Verification items for the finished model (mm, model axes). A direction names the side the tool comes from. Round coordinates to 2 decimals unless told otherwise and drop trailing zeros. Order: outer loops, then holes, each group sorted by start corner. A loop starts at its lowest first (then second) coordinate and runs counter-clockwise, first axis right, second up. Notation, with made-up numbers: M 30,-5 L 64,-5 A14 ccw 64,6 Z; hole C 50,84.25 d6. An arc over 180 degrees is marked long. Use one line per item in the form item = value. Start each with the question number.
Item 1: Cross-section at B-B on z = 3.75. Enter the section's corners in (x, y).
Item 2: Cross-section at A-A on x = 0. Enter the section's corners in (y, z), then the cut area to 3 significant figures.
Item 3: Release check for a two-part mould opening along Y. For faces 1 (the flat face through (-4, 4, -1)), 2 (the flat face through (0, 0, 13)), 3 (the flat face through (0, 5, -2.5)) record: +Y half, -Y half, draft (parallel to the pull), parting line (faces both ways), or undercut.
Item 4: Tool access check on faces 4 (the flat face through (0, 0, 15)), 5 (the flat face through (4, 4, -1)), 6 (the cylindrical face through (-1.2, -4.59, 9.05)), 7 (the cylindrical face through (0, -6, 12)). Record the directions out of +Z, -Z, +X, -X, +Y, -Y that give a thin tool (end or side, any length) a straight path to the whole face; none if there is none.
Item 5: Cross-section at D-D on z = -1.25. Enter the section's corners in (x, y).
Item 6: Go/stop test with flat-tipped pins: pin 1 Ø5 at (y, z) = (-1.5, 5.5) entering from -X; pin 2 Ø3 at (x, z) = (0, 9) entering from -Y; pin 3 Ø3 at (y, z) = (-5, 5.5) entering from -X. Record where each tip stops, or that it passes through.
Item 7: Cross-section at C-C on y = 0. Enter the section's corners in (x, z).
Item 8: Thickness scan on probe 1 along Y at (x, z) = (0, 1.2); probe 2 along Z at (x, y) = (0, -4.9). Record the ranges inside material, lowest first. Write a range as [from, to].
from build123d import *

# Parameters (mm, degrees)
F2_R      = 3.05
F3_DEPTH  = 13
F4_R      = 0.5
F5_R      = 1.2
F6_DEPTH  = 7
F7_R      = 1.5
F8_DEPTH  = 13
F10_DEPTH = 2.5
F11_DEPTH = 2.5
F13_DEPTH = 2.5


with BuildPart() as f1:
    # F0 (on Front) → F1 (revolve)
    with BuildSketch(Plane.XZ):
        Polygon((-5, 0), (0, 0), (0, 15), (-6.5, 15), (-6.5, 0), align=None)
    revolve(axis=Axis((0, 0, -3.6677676575), (0, 0, -1)))

    # F2 (on face) → F3 (cut)
    with BuildSketch(Plane(origin=(0, 0, 0), x_dir=(1, 0, 0), z_dir=(0, 0, -1))):
        Circle(F2_R)
    extrude(amount=-F3_DEPTH, mode=Mode.SUBTRACT)

    # F4
    f4_edges = [f1.edges().sort_by_distance(p)[0] for p in [
        (6.5, 0, 15),
    ]]
    fillet(f4_edges, radius=F4_R)

    # F5 (on Front) → F6 (cut)
    with BuildSketch(Plane.XZ):
        with Locations((0, 9)):
            Circle(F5_R)
    extrude(amount=F6_DEPTH, mode=Mode.SUBTRACT)

    # F7 (on face) → F8 (cut)
    with BuildSketch(Plane(origin=(0, 0, 0), x_dir=(1, 0, 0), z_dir=(0, 0, -1))):
        with Locations((-7.5, 0)):
            Circle(F7_R)
        with Locations((-6.4951905284, -3.75)):
            Circle(F7_R)
        with Locations((-3.75, -6.4951905284)):
            Circle(F7_R)
        with Locations((0, -7.5)):
            Circle(F7_R)
        with Locations((3.75, -6.4951905284)):
            Circle(F7_R)
        with Locations((6.4951905284, -3.75)):
            Circle(F7_R)
        with Locations((7.5, 0)):
            Circle(F7_R)
        with Locations((6.4951905284, 3.75)):
            Circle(F7_R)
        with Locations((3.75, 6.4951905284)):
            Circle(F7_R)
        with Locations((0, 7.5)):
            Circle(F7_R)
        with Locations((-3.75, 6.4951905284)):
            Circle(F7_R)
        with Locations((-6.4951905284, 3.75)):
            Circle(F7_R)
    extrude(amount=-F8_DEPTH, mode=Mode.SUBTRACT)

    # F9 (on face) → F10 (cut)
    with BuildSketch(Plane(origin=(0, 0, 0), x_dir=(1, 0, 0), z_dir=(0, 0, -1))):
        with BuildLine():
            Line((-5.6568542495, -5.6568542495), (0, 0))
            Line((0, 0), (5.6568542495, -5.6568542495))
            ThreePointArc((5.6568542495, -5.6568542495), (0, 8), (-5.6568542495, -5.6568542495))
        make_face()
    extrude(amount=-F10_DEPTH, mode=Mode.SUBTRACT)

    # F11 (add): faces of the model
    f11_faces = [f1.faces().sort_by_distance(p)[0] for p in [
        (-4.6979425412, 4.2437625345, 2.5),
        (0, 4.3753680924, 0),
    ]]
    extrude(f11_faces, amount=F11_DEPTH)

    # F12 (on face) → F13 (cut)
    with BuildSketch(Plane(origin=(0, 0, -2.5), x_dir=(1, 0, 0), z_dir=(0, 0, -1))):
        with BuildLine():
            ThreePointArc((2.1566756826, -2.1566756826), (0, -3.05), (-2.1566756826, -2.1566756826))
            Line((-2.1566756826, -2.1566756826), (-2.8637824638, -2.8637824638))
            ThreePointArc((-2.8637824638, -2.8637824638), (0, -4.0711582499), (2.8637824638, -2.8637824638))
            Line((2.8637824638, -2.8637824638), (2.1566756826, -2.1566756826))
        make_face()
    extrude(amount=-F13_DEPTH, mode=Mode.SUBTRACT)


solid = f1.part
Output values:
q1.outline = M -6.42,-1.04 A6.5 ccw -6.08,-2.31 A1.5 cw -5.04,-4.11 A6.5 ccw -4.11,-5.04 A1.5 cw -2.31,-6.08 A6.5 ccw -1.04,-6.42 A1.5 cw 1.04,-6.42 A6.5 ccw 2.31,-6.08 A1.5 cw 4.11,-5.04 A6.5 ccw 5.04,-4.11 A1.5 cw 6.08,-2.31 A6.5 ccw 6.42,-1.04 A1.5 cw 6.42,1.04 A6.5 ccw 6.08,2.31 A1.5 cw 5.04,4.11 A6.5 ccw 4.11,5.04 A1.5 cw 2.31,6.08 A6.5 ccw 1.04,6.42 A1.5 cw -1.04,6.42 A6.5 ccw -2.31,6.08 A1.5 cw -4.11,5.04 A6.5 ccw -5.04,4.11 A1.5 cw -6.08,2.31 A6.5 ccw -6.42,1.04 A1.5 cw Z; hole C 0,0 d6.1
q2.outline = M -6.5,13 L -6,13 L -6,10.2 L -3.05,10.2 L -3.05,13 L 3.05,13 L 3.05,0 L 4.07,0 L 4.07,-2.5 L 6,-2.5 L 6,13 L 6.5,13 L 6.5,14.5 A0.5 ccw 6,15 L -6,15 A0.5 ccw -6.5,14.5 Z; M -6,0 L -3.05,0 L -3.05,7.8 L -6,7.8 Z
q2.area = 100 mm2
q3.face_1 = -Y half
q3.face_2 = undercut
q3.face_3 = draft
q4.face_4 = +Z, +X, -X, +Y, -Y
q4.face_5 = -Z, +X, -Y
q4.face_6 = -Y
q4.face_7 = -Z, -Y
q5.outline = M -4.6,4.6 L -2.86,2.86 A4 cw 2.86,2.86 L 4.6,4.6 A6.5 ccw 4.11,5.04 A1.5 cw 2.31,6.08 A6.5 ccw 1.04,6.42 A1.5 cw -1.04,6.42 A6.5 ccw -2.31,6.08 A1.5 cw -4.11,5.04 A6.5 ccw Z
q6.pin_1 = -6.42
q6.pin_2 = -6.42
q6.pin_3 = -5.04
q7.outline = M -6.5,13 L -6,13 L -6,0 L -3.05,0 L -3.05,13 L 3.05,13 L 3.05,0 L 6,0 L 6,13 L 6.5,13 L 6.5,14.5 A0.5 ccw 6,15 L -6,15 A0.5 ccw -6.5,14.5 Z
q8.probe_1 = [-6, -3.05], [3.05, 6]
q8.probe_2 = [0, 7.8], [10.2, 15]
